Source: three-view drawing plus pictorial views. Frame: mm from the lowest corner of the part. A direction names the side the tool comes from. Coordinates: 2 decimals unless noted, no trailing zeros. Loops run counter-clockwise (first coordinate to the right, second up) from the corner with the lowest first, then second, coordinate; pieces in that order, holes last. Notation, with made-up numbers: (8.5, 11) - (63.5, 11) arc R20 ccw to (63.5, 18) - close; hole circle Ø10 at (-38.75, 81). An arc over 180 degrees is marked (long way). Return JSON: item names as keys, results as strings.
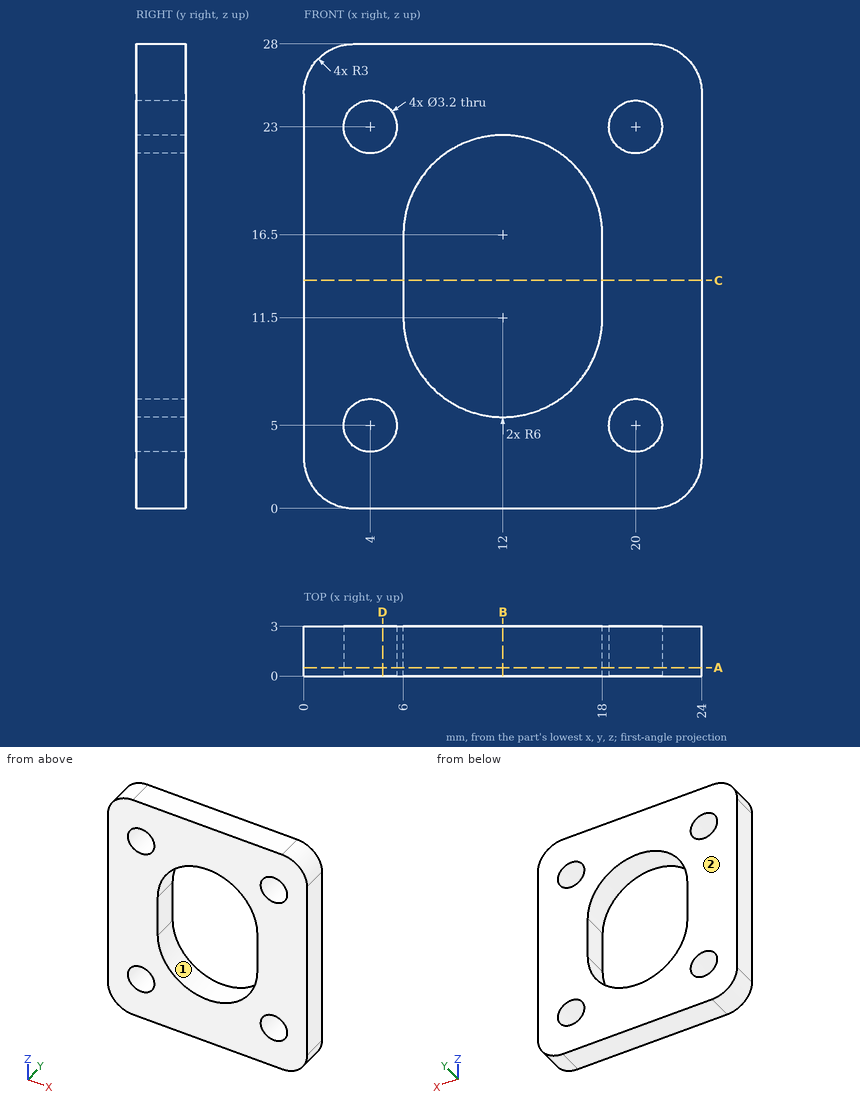
Item 1: First-contact query: pin 1 Ø2.5 at (x, z) = (4, 23) entering from -Y. Flat tip, straight axial feed; report the tip coordinate or a pass-through.
Worked out:
{"pin 1": "through"}
Item 2: Section query D-D, the plane x = 4.75. Return loops of the section in (y, z).
Worked out:
{"outline": "(0, 0) - (3, 0) - (3, 3.59) - (0, 3.59) - close; (0, 6.41) - (3, 6.41) - (3, 21.59) - (0, 21.59) - close; (0, 24.41) - (3, 24.41) - (3, 28) - (0, 28) - close"}
Item 3: Section query B-B, the plane x = 12. Return loops of the section in (y, z).
Worked out:
{"outline": "(0, 0) - (3, 0) - (3, 5.5) - (0, 5.5) - close; (0, 22.5) - (3, 22.5) - (3, 28) - (0, 28) - close"}
Item 4: Section query A-A, the plane y = 0.5. Return loops of the section in (x, z), and give its area (3 significant figures).
Worked out:
{"outline": "(0, 3) arc R3 ccw to (3, 0) - (21, 0) arc R3 ccw to (24, 3) - (24, 25) arc R3 ccw to (21, 28) - (3, 28) arc R3 ccw to (0, 25) - close; hole circle Ø3.2 at (4, 5); hole circle Ø3.2 at (4, 23); hole (6, 11.5) arc R6 ccw to (18, 11.5) - (18, 16.5) arc R6 ccw to (6, 16.5) - close; hole circle Ø3.2 at (20, 5); hole circle Ø3.2 at (20, 23)", "area": "459 mm^2"}
Item 5: Reachability of the marked faces 1 and 2 from +Z, -Z, +X, -X, +Y, -Y: full face, straight path, thin tool, end or side. Return the list, or none.
Worked out:
{"face 1": "+Y, -Y", "face 2": "+Z, -Z, +X, -X, +Y"}
Item 6: Section query C-C, the plane z = 13.75. Return loops of the section in (x, y).
Worked out:
{"outline": "(0, 0) - (6, 0) - (6, 3) - (0, 3) - close; (18, 0) - (24, 0) - (24, 3) - (18, 3) - close"}
Item 7: Ray query, probe 1 along X at (y, z) = (2.1, 23); probe 2 along X at (y, z) = (1.1, 16.75); probe 3 along X at (y, z) = (1.05, 6). Return the intervals inside material, ascending. Write a range as from..to.
Worked out:
{"probe 1": "0..2.4, 5.6..18.4, 21.6..24", "probe 2": "0..6.01, 17.99..24", "probe 3": "0..2.75, 5.25..9.6, 14.4..18.75, 21.25..24"}
